Model file for the job. Use its own axes, mm. A direction names the side the tool comes from. Round coordinates to 2 decimals unless told otherwise and drop trailing zeros. Order: outer loops, then holes, each group sorted by start corner. A loop starts at its lowest first (then second) coordinate and runs counter-clockwise, first axis right, second up. Notation, with made-up numbers: M -0.75,5 L 47.25,5 A27 ccw 47.25,44 Z; hole C 37,2.5 d7. An arc over 180 degrees is marked long. Return JSON: item names as keys, results as strings. Group by question number.
Item 1: Pin check, flat tips, straight feed: pin 1 Ø10 at (x, z) = (3, 9) entering from +Y; pin 2 Ø1.5 at (x, y) = (6.5, 4.5) entering from +Z; pin 3 Ø2 at (y, z) = (6.5, 8.5) entering from +X; pin 4 Ø1 at (y, z) = (2.5, 11) entering from +X. Stop position of each tip, or through.
Item 2: Slice it at C-C on z = 13.5. Write the cut outline in (x, y).
Item 3: Probe line 1 along Y through (x, z) = (-4.75, 12); line 2 along Z through (x, y) = (-4.75, 4); line 3 along X through (y, z) = (7.5, -1). List the from-to ranges inside material, lowest first.
Item 4: Which spindle directions (+Z, -Z, +X, -X, +Y, -Y) get a long thin tool onto all of the face, cutting with end or side? Do faces 5 (the face through (-4, 3.9, 14.2)), 6 (the face through (-9, 4, 7)). Say none if no direction does.
Item 5: Slice it at A-A on y = 4. Write the cut outline in (x, z), then the cut area to 3 significant figures.
Item 6: Slice it at B-B on x = -5. Write the cut outline in (y, z), then the cut area to 3 significant figures.
Item 7: Pull direction Y, two halves, no side cores. Call faces 1 (the face through (-4, 8, 5)), 2 (the face through (1.802, 3.944, 5.723)), 3 (the face through (-7, 4, 10)), 4 (the face through (-4, 0, 5)): pulls with the +Y half, pulls with the -Y half, needs draft (parallel to the pull), parting line crosses it, or undercut.
Item 8: Slice it at D-D on y = 0.75. Write the cut outline in (x, z).
from build123d import *

# Parameters (mm, degrees)
CROQUIS1_R              = 6
SALIENTE_EXTRUIR1_DEPTH = 8
CROQUIS3_R              = 2
CORTAR_EXTRUIR1_DEPTH   = 10


with BuildPart() as part:
    # Croquis1 → Saliente-Extruir1 (new body)
    with BuildSketch(Plane(origin=(0, 0, 0), x_dir=(1, 0, 0), z_dir=(0, 1, 0))):
        with BuildLine():
            Line((-9, 0), (-9, -15))
            Line((-9, -15), (-4, -15))
            Line((-4, -15), (-4, -13))
            ThreePointArc((-4, -13), (-2.828427125, -10.171572875), (0, -9))
            ThreePointArc((0, -9), (6.363961031, 6.363961031), (-9, 0))
        make_face()
        with Locations(Location((0, 0, 0), (0, 0, 270))):
            Circle(CROQUIS1_R, mode=Mode.SUBTRACT)
    extrude(amount=SALIENTE_EXTRUIR1_DEPTH)

    # Croquis3 → Cortar-Extruir1 (cut)
    with BuildSketch(Plane.ZY.offset(9)):
        with Locations((12, 4)):
            Circle(CROQUIS3_R)
    extrude(amount=-CORTAR_EXTRUIR1_DEPTH, mode=Mode.SUBTRACT)


solid = part.part
Output values:
{
 "1": {"pin 1": "y = 8", "pin 2": "z = 6.92", "pin 3": "x = 4.97", "pin 4": "x = -3.12"},
 "2": {"outline": "M -9,0 L -4,0 L -4,2.68 L -9,2.68 Z; M -9,5.32 L -4,5.32 L -4,8 L -9,8 Z"},
 "3": {"line 1": "0 to 2, 6 to 8", "line 2": "-7.64 to -3.67, 3.67 to 10, 14 to 15", "line 3": "-8.94 to -5.92, 5.92 to 8.94"},
 "4": {"face 5": "+Z, +X, +Y, -Y", "face 6": "+Z, -Z, -X, +Y, -Y"},
 "5": {"outline": "M -9,0 A9 ccw long 0,9 A4 cw -2.65,10 L -9,10 Z; M -9,14 L -4,14 L -4,15 L -9,15 Z; hole C 0,0 d12", "area": "171 mm²"},
 "6": {"outline": "M 0,-7.48 L 8,-7.48 L 8,-3.32 L 0,-3.32 Z; M 0,3.32 L 8,3.32 L 8,15 L 0,15 Z; hole C 4,12 d4", "area": "114 mm²"},
 "7": {"face 1": "pulls with the +Y half", "face 2": "needs draft", "face 3": "undercut", "face 4": "pulls with the -Y half"},
 "8": {"outline": "M -9,0 A9 ccw long 0,9 A4 cw -4,13 L -4,15 L -9,15 Z; hole C 0,0 d12"}
}
